Can you work these out from the model? Positions are in its coordinate system, mm. A direction names the side the tool comes from. Give positions to 0.01 mm unless a question says otherwise; leave off trailing zeros. Order: outer loops, then holes, each group sorted by start corner. A loop starts at its lowest first (then second) coordinate and runs counter-clockwise, first axis right, second up. Notation, with made-up numbers: (-20.5, 58.25) - (-13.5, 58.25) arc R7 ccw to (-13.5, 62.25) - close; hole circle Ø11 at (13.5, 56). An arc over 180 degrees is marked (long way). Answer as CSV lines item,"result".
```python
from build123d import *

# Parameters (mm, degrees)
F0_W     = 304.8
F0_H     = 152.4
F1_DEPTH = 6.35
F3_DEPTH = 6.35
F5_DEPTH = 25.399999693
F6_DEPTH = 25.4


with BuildPart() as f1:
    # F0 (on Right) → F1 (new body)
    with BuildSketch(Plane.YZ):
        Rectangle(F0_W, F0_H)
    extrude(amount=F1_DEPTH)

    # F2 (on face) → F3 (join)
    with BuildSketch(Plane.YZ.offset(6.35)):
        Polygon((-152.4, -76.2), (152.4, -76.2), (152.4, 0), (0, 76.2), (-152.4, 76.2), align=None)
    extrude(amount=F3_DEPTH)

    # F4 (on face) → F5 (join)
    with BuildSketch(Plane(origin=(0, 0, 0), x_dir=(0, -1, 0), z_dir=(-1, 0, 0))):
        Polygon((-152.4, 76.2), (-152.4, 0), (0, 76.2), align=None)
    extrude(amount=-F5_DEPTH)

    # F6 (add): a face of the model
    f6_faces = [f1.faces().sort_by_distance(p)[0] for p in [
        (0, 0, 0),
    ]]
    extrude(f6_faces, amount=F6_DEPTH)


solid = f1.part
```
1) I need wall thicknesses on line 1 along X through (y, z) = (-101.5, -65); line 2 along Z through (x, y) = (21, 124); line 3 along Y through (x, z) = (15, 27). Which ranges of each line are inside material? Lowest first, please. Write a range as [from, to].
Answer block:
line 1,"[-25.4, 12.7]"
line 2,"[14.2, 76.2]"
line 3,"[98.4, 152.4]"
2) I want a section at A-A on y = 10. Write out the boundary of the cut face in (x, z).
Answer block:
outline,"(-25.4, -76.2) - (12.7, -76.2) - (12.7, 71.2) - (25.4, 71.2) - (25.4, 76.2) - (-25.4, 76.2) - close"
3) I'm going to push a flat-ended pin straight in: P1, Ø12, axis at y = -19, z = -32.5, coming from the +X side. Where does the tip first touch, or does it pass through?
Answer block:
P1,"x = 12.7"
4) I want a section at C-C on y = -121. Write out the boundary of the cut face in (x, z), plus the area to 3 significant figures.
Answer block:
outline,"(-25.4, -76.2) - (12.7, -76.2) - (12.7, 76.2) - (-25.4, 76.2) - close"
area,"5,810 mm2"
5) I want a section at B-B on z = 15. Write out the boundary of the cut face in (x, y), plus the area to 3 significant figures.
Answer block:
outline,"(-25.4, -152.4) - (12.7, -152.4) - (12.7, 122.4) - (25.4, 122.4) - (25.4, 152.4) - (-25.4, 152.4) - close"
area,"12,000 mm2"
6) Which directions (+Z, -Z, +X, -X, +Y, -Y) give clear straight access to the entire face, cutting with the end or side of a thin tool? Please do faces 1 (the flat face through (12.7, -2, 1)), 2 (the flat face through (25.4, 94, 47)).
Answer block:
face 1,"-Z, +X, -Y"
face 2,"+Z, -Z, +X, +Y, -Y"
7) I want a section at D-D on z = -40. Write out the boundary of the cut face in (x, y).
Answer block:
outline,"(-25.4, -152.4) - (12.7, -152.4) - (12.7, 152.4) - (-25.4, 152.4) - close"
